Work out the finished part from the listing and answer in its coordinate system (mm). A direction names the side the tool comes from. Round coordinates to 2 decimals unless told otherwise and drop trailing zeros. Use one line per item in the form item = value.
```python
from build123d import *

# Parameters (mm, degrees)
SKETCH1_W                                           = 180
SKETCH1_H                                           = 130
BOSS_EXTRUDE1_DEPTH                                 = 10
CSK_FOR_M4_COUNTERSUNK_FLAT_HEAD_SCREW1_D           = 4.5
CSK_FOR_M4_COUNTERSUNK_FLAT_HEAD_SCREW1_DEPTH       = 6
CSK_FOR_M4_COUNTERSUNK_FLAT_HEAD_SCREW1_CSINK_D     = 9.4
CSK_FOR_M4_COUNTERSUNK_FLAT_HEAD_SCREW1_CSINK_ANGLE = 90
CSK_FOR_M4_COUNTERSUNK_FLAT_HEAD_SCREW1_TIP         = 1.351936393


with BuildPart() as part:
    # Sketch1 → Boss-Extrude1 (new body)
    with BuildSketch(Plane.XY):
        with Locations((90, 65)):
            Rectangle(SKETCH1_W, SKETCH1_H)
    extrude(amount=BOSS_EXTRUDE1_DEPTH)

    # CSK for M4 Countersunk Flat Head Screw1
    with Locations(Plane.XY.offset(10)):
        with Locations((10, 100), (40, 100), (10, 30), (40, 30), (140, 100), (170, 100), (140, 30), (170, 30)):
            CounterSinkHole(CSK_FOR_M4_COUNTERSUNK_FLAT_HEAD_SCREW1_D / 2, CSK_FOR_M4_COUNTERSUNK_FLAT_HEAD_SCREW1_CSINK_D / 2, depth=CSK_FOR_M4_COUNTERSUNK_FLAT_HEAD_SCREW1_DEPTH, counter_sink_angle=CSK_FOR_M4_COUNTERSUNK_FLAT_HEAD_SCREW1_CSINK_ANGLE)
            with Locations((0, 0, -(CSK_FOR_M4_COUNTERSUNK_FLAT_HEAD_SCREW1_DEPTH + CSK_FOR_M4_COUNTERSUNK_FLAT_HEAD_SCREW1_TIP / 2))):  # 118° drill point
                Cone(0, CSK_FOR_M4_COUNTERSUNK_FLAT_HEAD_SCREW1_D / 2, CSK_FOR_M4_COUNTERSUNK_FLAT_HEAD_SCREW1_TIP, mode=Mode.SUBTRACT)


solid = part.part
```
(1) For faces 1 (the cylindrical face through (10.488, 97.804, 5.75)), 2 (the flat face through (89, 0, 5)), determine the directions among +Z, -Z, +X, -X, +Y, -Y from which every point of the face is accessible in a straight line to the end or side of a thin tool.
Completed:
face_1 = +Z
face_2 = +Z, -Z, +X, -X, -Y
(2) Consider L1, parallel to X at y = 30, z = 6.75; L2, parallel to Y at x = 170, z = 5.6; L3, parallel to X at y = 103.5, z = 9.25. Determine where each line is inside the solid, lowest interval first.
Completed:
L1 = 0 to 7.75, 12.25 to 37.75, 42.25 to 137.75, 142.25 to 167.75, 172.25 to 180
L2 = 0 to 27.75, 32.25 to 97.75, 102.25 to 130
L3 = 0 to 8.17, 11.83 to 38.17, 41.83 to 138.17, 141.83 to 168.17, 171.83 to 180
(3) For a pull along X with two mould halves and no side action, classify faces 3 (the flat face through (180, 64, 5)), 4 (the flat face through (89, 130, 5)), 5 (the conical face through (41.88, 28.56, 7.67)) as +X half, -X half, draft (parallel to the pull), parting line (faces both ways), or undercut.
Completed:
face_3 = +X half
face_4 = draft
face_5 = undercut
(4) Given P1, Ø7, axis at x = 10, y = 100, coming from the -Z side; P2, Ø4, axis at x = 170, y = 30, coming from the +Z side; P3, Ø7, axis at x = 40, y = 100, coming from the +Z side; P4, Ø2.5, axis at x = 140, y = 100, coming from the +Z side, each flat-ended and moving along its own axis, determine where each tip first touches the part or whether it passes through.
Completed:
P1 = 0
P2 = 3.85
P3 = 8.8
P4 = 3.4
